```python
from build123d import *

# Parameters (mm, degrees)
SKETCH1_W           = 20.5
SKETCH1_H           = 16.25
SKETCH1_R           = 1.625
BOSS_EXTRUDE1_DEPTH = 1.6
FILLET1_R           = 1
SKETCH2_W           = 2.5
SKETCH2_H           = 8
BOSS_EXTRUDE2_DEPTH = 2.5
FILLET2_R           = 0.5
SKETCH8_W           = 0.55
SKETCH8_H           = 0.55
SKETCH9_W           = 0.55
SKETCH9_H           = 0.55
SKETCH4_W           = 0.55
SKETCH4_H           = 0.55


with BuildPart() as part:
    # Sketch1 → Boss-Extrude1 (new body)
    with BuildSketch(Plane(origin=(0, 0, 0), x_dir=(1, 0, 0), z_dir=(0, 1, 0))):
        Rectangle(SKETCH1_W, SKETCH1_H)
        with Locations(Location((7.625, 5.7, 0), (0, 0, 270))):
            Circle(SKETCH1_R, mode=Mode.SUBTRACT)
        with Locations(Location((7.625, -5.7, 0), (0, 0, 90))):
            Circle(SKETCH1_R, mode=Mode.SUBTRACT)
    extrude(amount=BOSS_EXTRUDE1_DEPTH)

    # Fillet1
    fillet1_edges = [part.edges().sort_by_distance(p)[0] for p in [
        (10.25, 0.8, 8.125),
        (-10.25, 0.8, 8.125),
        (-10.25, 0.8, -8.125),
        (10.25, 0.8, -8.125),
    ]]
    fillet(fillet1_edges, radius=FILLET1_R)

    # Sketch2 → Boss-Extrude2 (add)
    with BuildSketch(Plane(origin=(0, 1.6, 0), x_dir=(1, 0, 0), z_dir=(0, 1, 0))):
        with Locations((-9, 0)):
            Rectangle(SKETCH2_W, SKETCH2_H)
    extrude(amount=BOSS_EXTRUDE2_DEPTH)

    # Fillet2
    fillet2_edges = [part.edges().sort_by_distance(p)[0] for p in [
        (-7.75, 2.85, 4),
        (-7.75, 2.85, -4),
        (-10.25, 2.85, -4),
        (-10.25, 2.85, 4),
    ]]
    fillet(fillet2_edges, radius=FILLET2_R)

    # Sweep2: sweep along a path in Sketch5
    with BuildLine(Plane.XY.offset(-2.5)) as sweep2_path:
        Line((-9, 4.1), (-9, 4.85))
        ThreePointArc((-9, 4.85), (-9.317041617, 5.34027213), (-9.839940826, 5.6))
        Line((-9.839940826, 5.6), (-17, 5.6))
    # Sketch8 → Sweep2 (sweep)
    with BuildSketch(Plane(origin=(0, 4.1, 0), x_dir=(1, 0, 0), z_dir=(0, 1, 0))):
        with Locations((-9.001105099, 2.502876889)):
            Rectangle(SKETCH8_W, SKETCH8_H)
    sweep(path=sweep2_path.line, transition=Transition.RIGHT)

    # Sweep3: sweep along a path in Sketch6
    with BuildLine(Plane.XY.offset(2.5)) as sweep3_path:
        Line((-9, 4.1), (-9, 4.85))
        ThreePointArc((-9, 4.85), (-9.317041617, 5.34027213), (-9.839940826, 5.6))
        Line((-9.839940826, 5.6), (-17, 5.6))
    # Sketch9 → Sweep3 (sweep)
    with BuildSketch(Plane(origin=(0, 4.1, 0), x_dir=(1, 0, 0), z_dir=(0, 1, 0))):
        with Locations((-8.999962547, -2.498553748)):
            Rectangle(SKETCH9_W, SKETCH9_H)
    sweep(path=sweep3_path.line, transition=Transition.RIGHT)

    # Sweep4: sweep along a path in Sketch3
    with BuildLine(Plane.XY) as sweep4_path:
        Line((-9, 4.1), (-9, 4.85))
        ThreePointArc((-9, 4.85), (-9.317041617, 5.34027213), (-9.839940826, 5.6))
        Line((-9.839940826, 5.6), (-17, 5.6))
    # Sketch4 → Sweep4 (sweep)
    with BuildSketch(Plane(origin=(0, 4.1, 0), x_dir=(1, 0, 0), z_dir=(0, 1, 0))):
        with Locations((-9, 0)):
            Rectangle(SKETCH4_W, SKETCH4_H)
    sweep(path=sweep4_path.line, transition=Transition.RIGHT)


solid = part.part
```
The listing builds one solid part. Answer for the finished solid, in the listing's coordinates (mm). A direction names the side the tool comes from. Round coordinates to 2 decimals unless told otherwise and drop trailing zeros. Loops run counter-clockwise (first coordinate to the right, second up) from the corner with the lowest first, then second, coordinate; pieces in that order, holes last. Notation, with made-up numbers: (-32.75, 58.25) -> (14.25, 58.25) arc R27 cw to (14.25, 86.25) -> close; hole circle Ø11 at (61, 58.25). An arc over 180 degrees is marked (long way). Use one line per item in the form item = value.
1. A tool of negligible diameter and unlimited length cuts with its end or side. For faces 1 (the flat face through (-12, 5.6, -2.228)), 2 (the flat face through (-11.9, 5.6, -2.778)), 3 (the flat face through (-12, 5.6, 2.774)), from which of +Z, -Z, +X, -X, +Y, -Y can it reach the whole face along a straight path? Write none if from no direction.
Answer key:
face_1 = +X, -X, +Y
face_2 = -Z, +X, -X, +Y
face_3 = +Z, +X, -X, +Y
2. The part is cut by section A-A on z = -5.7. Determine the outline of the cut face in (x, y), and give its area (3 significant figures).
Answer key:
outline = (-10.25, 0) -> (6, 0) -> (6, 1.6) -> (-10.25, 1.6) -> close; (9.25, 0) -> (10.25, 0) -> (10.25, 1.6) -> (9.25, 1.6) -> close
area = 27.6 mm²
3. The part is cut by section C-C on z = 5.5. Determine the outline of the cut face in (x, y), and give its area (3 significant figures).
Answer key:
outline = (-10.25, 0) -> (6.01, 0) -> (6.01, 1.6) -> (-10.25, 1.6) -> close; (9.24, 0) -> (10.25, 0) -> (10.25, 1.6) -> (9.24, 1.6) -> close
area = 27.6 mm²
4. Flat-ended cylindrical pins translate along their axes: pin 1 Ø2 at (x, y) = (-11.5, 5.5) entering from -Z; pin 2 Ø1 at (y, z) = (4, -4) entering from -X; pin 3 Ø0.6 at (x, z) = (-14, 2.5) entering from -Y. Find the tip coordinate at first contact, or state that the pin passes through.
Answer key:
pin_1 = -2.78
pin_2 = -10.25
pin_3 = 5.33
5. Find the intervals of material crossed by probe 1 along X at (y, z) = (0.45, -5.7); probe 2 along Z at (x, y) = (7.5, 0.8) (3 decimals); probe 3 along Y at (x, z) = (-0.5, 3.25), in increasing order. Write a range as [from, to].
Answer key:
probe_1 = [-10.25, 6], [9.25, 10.25]
probe_2 = [-8.125, -7.32], [-4.08, 4.08], [7.32, 8.125]
probe_3 = [0, 1.6]
6. The part is cut by section B-B on y = 2.85. Determine the outline of the cut face in (x, z).
Answer key:
outline = (-10.25, -3.5) arc R0.5 ccw to (-9.75, -4) -> (-8.25, -4) arc R0.5 ccw to (-7.75, -3.5) -> (-7.75, 3.5) arc R0.5 ccw to (-8.25, 4) -> (-9.75, 4) arc R0.5 ccw to (-10.25, 3.5) -> close
7. For a pull along Z with two mould halves and no side action, classify faces 4 (the cylindrical face through (9.236, 0.789, -5.912)), 5 (the flat face through (-9, 3, 4)), 6 (the flat face through (-10.25, 2, 0)) as released by +Z, released by -Z, zero draft, split by the parting line, or undercut.
Answer key:
face_4 = undercut
face_5 = released by +Z
face_6 = zero draft
8. The part is cut by section D-D on x = -4.75. Determine the outline of the cut face in (y, z) (3 decimals), and give its area (3 significant figures).
Answer key:
outline = (0, -8.125) -> (1.6, -8.125) -> (1.6, 8.125) -> (0, 8.125) -> close
area = 26.0 mm²
